For this review, take the finished solid that the model builds, in its own axes (mm). A direction names the side the tool comes from. Give positions to 0.01 mm unless a question says otherwise; leave off trailing zeros. Write each loop counter-clockwise with the first axis right and the second up, starting at its lowest first coordinate (ties: lowest second). Pieces come first, ordered by that corner, then holes.
1) For P1, Ø2, axis at x = -0.5, z = 0.5, coming from the +Y side; P2, Ø2, axis at y = -2, z = -5, coming from the -X side; P3, Ø0.5, axis at x = 0, z = -2.5, coming from the +Y side; P4, Ø6, axis at x = 5.5, y = -10.5, coming from the +Z side, all flat-tipped, find the tip position at first contact; note any pin that passes through.
2) Draft analysis for pull direction X (two halves, no side actions). For faces 4 (the face through (0, -0.2, 2)), 5 (the face through (6.21, -1.25, -3.23)), 6 (the face through (0, 0, 0)), state which applies: pulls with the +X half, pulls with the -X half, needs draft (parallel to the pull), parting line crosses it, or undercut.
3) Wall thickness on line 1 along X through (y, z) = (-0.1, 0); line 2 along Y through (x, z) = (1.5, 1.75); line 3 along Z through (x, y) = (-0.25, -9): over which ranges is each line inside the solid? List them lowest first.
4) Machinability: for faces 1 (the face through (0, -0.2, -2)), 2 (the face through (-4.5, 0, -1.4)), 3 (the face through (-1.802, -11.64, -5.723)), which of the approach directions +Z, -Z, +X, -X, +Y, -Y give a long, thin tool a straight path to every point of the face, cutting with its end or side? Answer none if there is none.
5) We need section B-B on z = 0. Give the boundary of the cut face in (x, y).
6) We need section A-A on x = 0. Give the boundary of the cut face in (y, z), and give its area (3 significant figures).
7) We need section C-C on y = -9.5. Give the boundary of the cut face in (x, z), and give its area (3 significant figures).
from build123d import *

# Parameters (mm, degrees)
FILLET_1_R          = 1
SKETCH_2_R          = 4.5
SKETCH_2_R_2        = 3.75
CUT_EXTRUDE_1_DEPTH = 0.2


with BuildPart() as part:
    # 草图1 → 旋转1 (revolve)
    with BuildSketch(Plane.XY, mode=Mode.PRIVATE) as revolve_1_sk:
        Polygon((0, 0), (7, 0), (7, -1.5), (6, -1.5), (6, -21.5), (0, -21.5), align=None)
    revolve(revolve_1_sk.sketch.rotate(Axis((0, 0, 0), (0, 1, 0)), 90), axis=Axis((0, 0, 0), (0, 1, 0)))

    # 圆角1
    fillet_1_edges = [part.edges().sort_by_distance(p)[0] for p in [
        (0, 0, 7),
    ]]
    fillet(fillet_1_edges, radius=FILLET_1_R)

    # 草图2 → 切除-拉伸1 (cut)
    # profile 1 of 3: a face of its own
    with BuildSketch(Plane(origin=(0, 0, 0), x_dir=(1, 0, 0), z_dir=(0, 1, 0))):
        with Locations(Location((0, 0, 0), (0, 0, 270))):
            Circle(SKETCH_2_R)
        with Locations(Location((0, 0, 0), (0, 0, 270))):
            Circle(SKETCH_2_R_2, mode=Mode.SUBTRACT)
    # profile 2 of 3: a face of its own
    with BuildSketch(Plane(origin=(0, 0, 0), x_dir=(1, 0, 0), z_dir=(0, 1, 0))):
        with BuildLine():
            ThreePointArc((-1.767766953, 1.767766953), (0, -2.5), (1.767766953, 1.767766953))
            ThreePointArc((1.767766953, 1.767766953), (1.060660172, 1.767766953), (1.060660172, 1.060660172))
            ThreePointArc((1.060660172, 1.060660172), (0, -1.5), (-1.060660172, 1.060660172))
            ThreePointArc((-1.060660172, 1.060660172), (-1.060660172, 1.767766953), (-1.767766953, 1.767766953))
        make_face()
    # profile 3 of 3: a face of its own
    with BuildSketch(Plane(origin=(0, 0, 0), x_dir=(1, 0, 0), z_dir=(0, 1, 0))):
        with BuildLine():
            Line((-0.5, 2.5), (-0.5, 1))
            ThreePointArc((-0.5, 1), (0, 0.5), (0.5, 1))
            Line((0.5, 1), (0.5, 2.5))
            ThreePointArc((0.5, 2.5), (0, 3), (-0.5, 2.5))
        make_face()
    extrude(amount=-CUT_EXTRUDE_1_DEPTH, mode=Mode.SUBTRACT)


solid = part.part
Results list:
1. P1: stops at y = 0
1. P2: stops at x = -5.65
1. P3: stops at y = -0.2
1. P4: stops at z = 5.45
2. face 4: undercut
2. face 5: parting line crosses it
2. face 6: needs draft
3. line 1: x = -6.44 to -4.5, -3.75 to -2.5, -1.5 to 1.5, 2.5 to 3.75, 4.5 to 6.44
3. line 2: y = -21.5 to -0.2
3. line 3: z = -5.99 to 5.99
4. face 1: +Y
4. face 2: +Z, -Z, +X, -X, +Y
4. face 3: -Y
5. outline: (-7, -1.5) - (-6, -1.5) - (-6, -21.5) - (6, -21.5) - (6, -1.5) - (7, -1.5) - (7, -1) arc R1 ccw to (6, 0) - (4.5, 0) - (4.5, -0.2) - (3.75, -0.2) - (3.75, 0) - (2.5, 0) - (2.5, -0.2) - (1.5, -0.2) - (1.5, 0) - (-1.5, 0) - (-1.5, -0.2) - (-2.5, -0.2) - (-2.5, 0) - (-3.75, 0) - (-3.75, -0.2) - (-4.5, -0.2) - (-4.5, 0) - (-6, 0) arc R1 ccw to (-7, -1) - close
6. outline: (-21.5, -6) - (-1.5, -6) - (-1.5, -7) - (-1, -7) arc R1 ccw to (0, -6) - (0, -4.5) - (-0.2, -4.5) - (-0.2, -3.75) - (0, -3.75) - (0, -3) - (-0.2, -3) - (-0.2, -0.5) - (0, -0.5) - (0, 1.5) - (-0.2, 1.5) - (-0.2, 2.5) - (0, 2.5) - (0, 3.75) - (-0.2, 3.75) - (-0.2, 4.5) - (0, 4.5) - (0, 6) arc R1 ccw to (-1, 7) - (-1.5, 7) - (-1.5, 6) - (-21.5, 6) - close
6. area: 260 mm2
7. outline: circle Ø12 at (0, 0)
7. area: 113 mm2
